from build123d import *

# Parameters (mm, degrees)
F0_W      = 50.8
F0_H      = 9.525
F1_DEPTH  = 3.175
F2_W      = 3.175
F2_H      = 9.525
F3_DEPTH  = 50.8
F4_W      = 4.7625
F4_H      = 4.7625
F5_DEPTH  = 12.7
F6_R      = 1.27
F7_W      = 9.525
F7_H      = 3.175
F8_DEPTH  = 3.175
F9_W      = 17.272898303
F9_H      = 3.175
F9_W_2    = 9.525
F10_DEPTH = 4.7625
F11_W     = 1.3907738797
F11_H     = 2.54
F12_DEPTH = 50.8
F13_R     = 0.635
F14_SIZE  = 3.17499


# Not quite as in the source:
# - a fillet or chamfer is up to 0.001 mm smaller than in the source, because OpenCascade refuses the exact size


with BuildPart() as f1:
    # F0 (on Front) → F1 (new body)
    with BuildSketch(Plane.XZ):
        Rectangle(F0_W, F0_H)
    extrude(amount=F1_DEPTH)

    # F2 (on face) → F3 (join)
    with BuildSketch(Plane.YZ.offset(25.4)):
        with Locations((-4.7625, 0)):
            Rectangle(F2_W, F2_H)
    extrude(amount=-F3_DEPTH)

    # F4 (on face) → F5 (join)
    with BuildSketch(Plane(origin=(0, 0, 0), x_dir=(-1, 0, 0), z_dir=(0, 1, 0))):
        with Locations((20.6375, 0)):
            Rectangle(F4_W, F4_H)
    extrude(amount=F5_DEPTH)

    # F6
    f6_edges = [f1.edges().sort_by_distance(p)[0] for p in [
        (-18.25625, 6.35, 2.38125),
        (-23.01875, 6.35, 2.38125),
        (-18.25625, 6.35, -2.38125),
        (-23.01875, 6.35, -2.38125),
    ]]
    fillet(f6_edges, radius=F6_R)

    # F7 (on face) → F8 (join)
    with BuildSketch(Plane.XY.offset(4.7625)):
        with Locations((12.889601697, -1.5875)):
            Rectangle(F7_W, F7_H)
    extrude(amount=F8_DEPTH)

    # F9 (on face) → F10 (join)
    with BuildSketch(Plane(origin=(0, 0, 0), x_dir=(-1, 0, 0), z_dir=(0, 1, 0))):
        with Locations((-16.7635508485, 3.175)):
            Rectangle(F9_W, F9_H)
        with Locations((-12.889601697, 6.35)):
            Rectangle(F9_W_2, F9_H)
    extrude(amount=F10_DEPTH)

    # F11 (on face) → F12 (cut)
    with BuildSketch(Plane.YZ.offset(25.4)):
        with Locations((-5.6546130601, 2.3944999478)):
            Rectangle(F11_W, F11_H)
        with Locations((-5.6546130601, -2.4159172396)):
            Rectangle(F11_W, F11_H)
    extrude(amount=-F12_DEPTH, mode=Mode.SUBTRACT)

    # F13
    f13_edges = [f1.edges().sort_by_distance(p)[0] for p in [
        (0, -4.959226, 1.1245),
        (0, -4.959226, 3.6645),
        (0, -4.959226, -3.685917),
        (0, -4.959226, -1.145917),
        (0, -6.35, 1.1245),
        (0, -6.35, -1.145917),
        (0, -6.35, 3.6645),
        (0, -6.35, -3.685917),
    ]]
    fillet(f13_edges, radius=F13_R)

    # F14 (size 3.175 in the source; OpenCascade refuses exactly that, so slightly less here)
    f14_edges = [f1.edges().sort_by_distance(p)[0] for p in [
        (12.889602, -3.175, 4.7625),
    ]]
    chamfer(f14_edges, length=F14_SIZE)


solid = f1.part
For this review, take the finished solid that the model builds, in its own axes (mm). A direction names the side the tool comes from. Round coordinates to 2 decimals unless told otherwise and drop trailing zeros. Loops run counter-clockwise (first coordinate to the right, second up) from the corner with the lowest first, then second, coordinate; pieces in that order, holes last. Notation, with made-up numbers: (27, -31) - (33, -31) arc R25 cw to (33, 8) - close; hole circle Ø9 at (79, 0.25). An arc over 180 degrees is marked (long way). Answer as CSV lines item,"result".
(1) Consider section D-D on y = 6.5. Give the boundary of the cut face in (x, z).
Checked values:
outline,"(-23.02, -1.11) arc R1.27 ccw to (-21.75, -2.38) - (-19.53, -2.38) arc R1.27 ccw to (-18.26, -1.11) - (-18.26, 1.11) arc R1.27 ccw to (-19.53, 2.38) - (-21.75, 2.38) arc R1.27 ccw to (-23.02, 1.11) - close"
(2) Mouldability with a two-part tool opening along Z and no side actions: class faces 1 (the face through (-22.637, 6.439, 2.019)), 2 (the face through (0, -4.959, 2)), 3 (the face through (-18.256, 6, 0)) as +Z half, -Z half, draft (parallel to the pull), parting line (faces both ways), or undercut.
Checked values:
face 1,"+Z half"
face 2,"undercut"
face 3,"draft"
(3) Tool access review of faces 4 (the face through (-21, 6, -2.381)), 5 (the face through (0, -3, 4.762)), 6 (the face through (-18.62, 6.44, 2)), 7 (the face through (-18.62, 6.44, -2)), 8 (the face through (-21, 6, 2.381)): name each direction out of +Z, -Z, +X, -X, +Y, -Y from which nothing blocks a thin tool from reaching the whole face with its end or side.
Checked values:
face 4,"-Z, +X, -X, +Y"
face 5,"+Z, -X, +Y, -Y"
face 6,"+Z, +Y"
face 7,"-Z, +X, +Y"
face 8,"+Z, -X, +Y"
(4) Wall thickness on line 1 (Z direction, x = -20.5, y = 4.25); line 2 (Y direction, x = 15, z = -2.75); line 3 (Z direction, x = 22, y = -1.75): over which ranges is each line inside the solid? List them lowest first.
Checked values:
line 1,"z = -2.38 to 2.38"
line 2,"y = -4.96 to 0"
line 3,"z = -4.76 to 4.76"
(5) Consider section A-A on y = -1.5. Give the boundary of the cut face in (x, z), then the cut area to 3 significant figures.
Checked values:
outline,"(-25.4, -4.76) - (25.4, -4.76) - (25.4, 4.76) - (17.65, 4.76) - (17.65, 7.94) - (8.13, 7.94) - (8.13, 4.76) - (-25.4, 4.76) - close"
area,"514 mm2"
(6) Insertion check: P1, Ø0.7, axis at y = 5.5, z = 0, coming from the +X side; P2, Ø3, axis at x = 15.5, z = 5.5, coming from the +Y side; P3, Ø1, axis at x = -14, z = -3, coming from the +Y side. Each pin has a flat end and moves straight along its axis. Give the tip position at first contact, or say it passes through.
Checked values:
P1,"stops at x = -18.26"
P2,"stops at y = 4.76"
P3,"stops at y = 0"
